```python
from build123d import *

# Parameters (mm, degrees)
CHAMFER1_SIZE      = 0.5
CUT_EXTRUDE1_DEPTH = 1.8


with BuildPart() as part:
    # Sketch1 → Revolve1 (revolve)
    with BuildSketch(Plane.XY, mode=Mode.PRIVATE) as revolve1_sk:
        Polygon((0, 180), (-6, 180), (-6, 149.25), (-5.75, 149.25), (-5.75, 148), (-6, 148), (-6, 0), (0, 0), align=None)
    revolve(revolve1_sk.sketch.rotate(Axis((0, 180, 0), (0, 1, 0)), 270), axis=Axis((0, 180, 0), (0, 1, 0)))

    # Chamfer1
    chamfer1_edges = [part.edges().sort_by_distance(p)[0] for p in [
        (0, 0, 6),
        (0, 180, 6),
    ]]
    chamfer(chamfer1_edges, length=CHAMFER1_SIZE)

    # Sketch2 → Cut-Extrude1 (cut)
    with BuildSketch(Plane.XY.offset(6)):
        with BuildLine():
            Line((-2, 160), (-2, 180))
            ThreePointArc((-2, 180), (0, 182), (2, 180))
            Line((2, 180), (2, 160))
            ThreePointArc((2, 160), (0, 158), (-2, 160))
        make_face()
    extrude(amount=-CUT_EXTRUDE1_DEPTH, mode=Mode.SUBTRACT)


solid = part.part
```
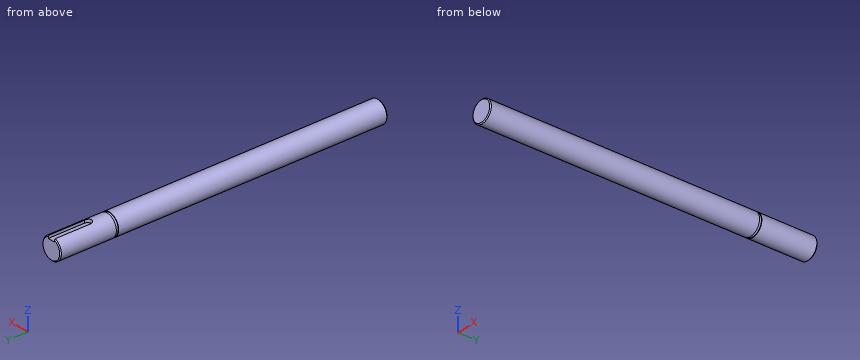
Could you check a few things on this model? Use its own coordinates, in mm. Give positions to 0.01 mm unless a question says otherwise; leave off trailing zeros. Loops run counter-clockwise (first coordinate to the right, second up) from the corner with the lowest first, then second, coordinate; pieces in that order, holes last. Notation, with made-up numbers: (-26.75, -36.75) - (21.25, -36.75) arc R13 ccw to (21.25, -17.75) - close; hole circle Ø9 at (-30.75, -18). An arc over 180 degrees is marked (long way). Use one line per item in the form item = value.
1. I want a section at B-B (y = 37.5). Please give me the cut outline in (x, z), and give its area (3 significant figures).
Response values:
outline = circle Ø12 at (0, 0)
area = 113 mm²
2. I want a section at C-C (y = 165). Please give me the cut outline in (x, z).
Response values:
outline = (-2, 4.2) - (-2, 5.66) arc R6 ccw (long way) to (2, 5.66) - (2, 4.2) - close
3. I'm going to push flat-ended pins straight in: pin 1 Ø3 at (y, z) = (34, -4.5) entering from -X; pin 2 Ø1.6 at (y, z) = (167, 5) entering from +X; pin 3 Ø1.5 at (y, z) = (110, -1) entering from -X. Where does each tip first touch, or does it pass through?
Response values:
pin_1 = -5.2
pin_2 = 4.28
pin_3 = -5.99
4. I want a section at A-A (x = 0). Please give me the cut outline in (y, z), and give its area (3 significant figures).
Response values:
outline = (0, -5.5) - (0.5, -6) - (148, -6) - (148, -5.75) - (149.25, -5.75) - (149.25, -6) - (179.5, -6) - (180, -5.5) - (180, 4.2) - (158, 4.2) - (158, 6) - (149.25, 6) - (149.25, 5.75) - (148, 5.75) - (148, 6) - (0.5, 6) - (0, 5.5) - close
area = 2,120 mm²
5. I need wall thicknesses on probe 1 along X at (y, z) = (139.5, 0.5); probe 2 along Z at (x, y) = (-1.75, 45.5); probe 3 along Z at (x, y) = (2.25, 122). Which ranges of each line are inside material? Lowest first, please.
Response values:
probe_1 = -5.98 to 5.98
probe_2 = -5.74 to 5.74
probe_3 = -5.56 to 5.56
